The figure shows three views and two pictorial views of one solid part (mm, origin at its lowest corner). Answer the questions. Coordinates: 2 decimals unless noted, no trailing zeros. Order: outer loops, then holes, each group sorted by start corner. A loop starts at its lowest first (then second) coordinate and runs counter-clockwise, first axis right, second up.
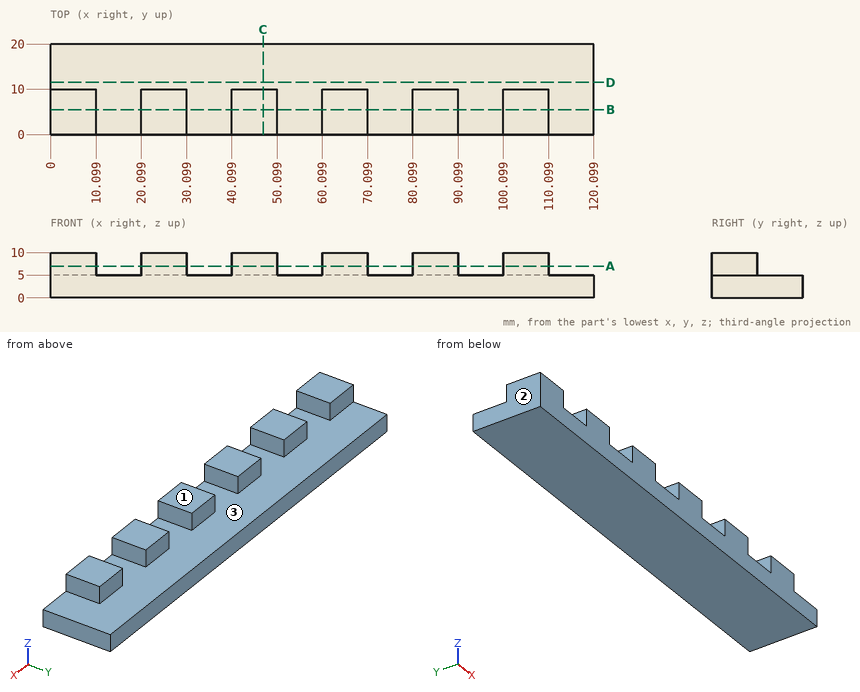
Q1. Each of these flat-tipped pins is pushed along its axis until it touches: P1, Ø2.5, axis at y = 6, z = 7, coming from the +X side; P2, Ø2.5, axis at x = 45, z = 8.5, coming from the +Y side; P3, Ø4, axis at y = 13.5, z = 8, coming from the -X side. Where does it stop, or does it pass through?
Q2. Straight lines are drawn through the part: L1, parallel to X at y = 7, z = 5.5; L2, parallel to Z at x = 102.5, y = 10.75; L3, parallel to Y at x = 42.5, z = 6.75. For each, find the intervals that lie inside material, in ascending order.
Q3. The part is cut by section B-B, the plane y = 5.5. Determine the outline of the cut face in (x, z), then the cut area to 3 significant figures.
Q4. The part is cut by section D-D, the plane y = 11.5. Determine the outline of the cut face in (x, z).
Q5. The part is cut by section C-C, the plane x = 47. Determine the outline of the cut face in (y, z), then the cut area to 3 significant figures.
Q6. The part is cut by section A-A, the plane z = 7. Determine the outline of the cut face in (x, y).
Q7. Determine the mould class of the marked faces 1, 2 and 3 for opening direction X: +X half, -X half, draft (parallel to the pull), parting line (faces both ways), or undercut.
Computed values:
1. P1: stops at x = 110.1
1. P2: stops at y = 10
1. P3: passes through
2. L1: x = 0 to 10.1, 20.1 to 30.1, 40.1 to 50.1, 60.1 to 70.1, 80.1 to 90.1, 100.1 to 110.1
2. L2: z = 0 to 5
2. L3: y = 0 to 10
3. outline: (0, 0) - (120.1, 0) - (120.1, 5) - (110.1, 5) - (110.1, 10) - (100.1, 10) - (100.1, 5) - (90.1, 5) - (90.1, 10) - (80.1, 10) - (80.1, 5) - (70.1, 5) - (70.1, 10) - (60.1, 10) - (60.1, 5) - (50.1, 5) - (50.1, 10) - (40.1, 10) - (40.1, 5) - (30.1, 5) - (30.1, 10) - (20.1, 10) - (20.1, 5) - (10.1, 5) - (10.1, 10) - (0, 10) - close
3. area: 901 mm2
4. outline: (0, 0) - (120.1, 0) - (120.1, 5) - (0, 5) - close
5. outline: (0, 0) - (20, 0) - (20, 5) - (10, 5) - (10, 10) - (0, 10) - close
5. area: 150 mm2
6. outline: (0, 0) - (10.1, 0) - (10.1, 10) - (0, 10) - close; (20.1, 0) - (30.1, 0) - (30.1, 10) - (20.1, 10) - close; (40.1, 0) - (50.1, 0) - (50.1, 10) - (40.1, 10) - close; (60.1, 0) - (70.1, 0) - (70.1, 10) - (60.1, 10) - close; (80.1, 0) - (90.1, 0) - (90.1, 10) - (80.1, 10) - close; (100.1, 0) - (110.1, 0) - (110.1, 10) - (100.1, 10) - close
7. face 1: draft
7. face 2: -X half
7. face 3: undercut
